Here's how the part is built. I have some questions about the finished solid (model axes, mm). A direction names the side the tool comes from. Coordinates: 2 decimals unless noted, no trailing zeros. Write each loop counter-clockwise with the first axis right and the second up, starting at its lowest first coordinate (ties: lowest second). Pieces come first, ordered by that corner, then holes.
Item 1: I want a section at A-A (x = 0). Please give me the cut outline in (y, z), and give its area (3 significant figures).
Item 2: I want a section at C-C (z = -19). Please give me the cut outline in (x, y), and give its area (3 significant figures).
Item 3: Please list where these lines run through material, in increasing order: line 1 (X direction, y = 1.2, z = 0); line 2 (X direction, y = 2.25, z = -4); line 3 (Y direction, x = -31, z = -31).
Item 4: I want a section at B-B (z = 0). Please give me the cut outline in (x, y), and give its area (3 significant figures).
Item 5: I'm going to push flat-ended pins straight in: P1, Ø5, axis at x = 28.5, z = 23, coming from the -Y side; P2, Ø2, axis at x = -18, y = 4, coming from the -Z side; P3, Ø1.5, axis at y = 1.5, z = -2, coming from the +X side. Where does each tip first touch, or does it pass through?
Item 6: For faces 1 (the face through (18.44, 3.166, -34.934)), 2 (the face through (19, 7.62, -33)), which set-ups out of +Z, -Z, +X, -X, +Y, -Y let a thin tool reach every point of the face, with its end or its side?
Item 7: I want a section at D-D (y = 6.25). Please give me the cut outline in (x, z), and give its area (3 significant figures).
from build123d import *

# Parameters (mm, degrees)
SKETCH1_R           = 44.45
SKETCH1_R_2         = 31.75
BOSS_EXTRUDE1_DEPTH = 2.54
CIRPATTERN1_COUNT   = 3


with BuildPart() as part:
    # Sketch1 → Boss-Extrude1 (new body)
    with BuildSketch(Plane(origin=(0, 0, 0), x_dir=(1, 0, 0), z_dir=(0, 1, 0))):
        with Locations(Location((0, 0, 0), (0, 0, 270))):
            Circle(SKETCH1_R)
        with Locations(Location((0, 0, 0), (0, 0, 270))):
            Circle(SKETCH1_R_2, mode=Mode.SUBTRACT)
    extrude(amount=BOSS_EXTRUDE1_DEPTH)

    # Sketch4 → Revolve1 (revolve)
    with BuildSketch(Plane.XY, mode=Mode.PRIVATE) as revolve1_sk:
        Polygon((-38.1, 2.54), (-38.1, 7.62), (-39.878, 7.62), (-40.132, 3.81), (-40.132, 2.54), align=None)
    revolve1 = revolve(revolve1_sk.sketch.rotate(Axis((-38.1, 2.54, 0), (0, 1, 0)), 270), axis=Axis((-38.1, 2.54, 0), (0, 1, 0)))

    # CirPattern1: Revolve1 ×3 about axis
    cirpattern1_axis = Axis((0, 0, 0), (0, 1, 0))
    for i in range(1, CIRPATTERN1_COUNT):
        add(revolve1.rotate(cirpattern1_axis, i * 360 / CIRPATTERN1_COUNT))


solid = part.part
Answer:
1. outline: (0, -44.45) - (2.54, -44.45) - (2.54, -31.75) - (0, -31.75) - close; (0, 31.75) - (2.54, 31.75) - (2.54, 44.45) - (0, 44.45) - close
1. area: 64.5 mm2
2. outline: (-40.18, 0) - (-25.44, 0) - (-25.44, 2.54) - (-40.18, 2.54) - close; (25.44, 0) - (40.18, 0) - (40.18, 2.54) - (25.44, 2.54) - close
2. area: 74.9 mm2
3. line 1: x = -44.45 to -31.75, 31.75 to 44.45
3. line 2: x = -44.27 to -31.5, 31.5 to 44.27
3. line 3: y = 0 to 2.54
4. outline: (-44.45, 0) - (-31.75, 0) - (-31.75, 2.54) - (-36.07, 2.54) - (-36.07, 3.81) - (-36.32, 7.62) - (-39.88, 7.62) - (-40.13, 3.81) - (-40.13, 2.54) - (-44.45, 2.54) - close; (31.75, 0) - (44.45, 0) - (44.45, 2.54) - (31.75, 2.54) - close
4. area: 84.2 mm2
5. P1: stops at y = 0
5. P2: passes through
5. P3: stops at x = 44.43
6. face 1: +Y
6. face 2: +Z, -Z, +X, -X, +Y
7. outline: circle Ø3.74 at (-38.1, 0); circle Ø3.74 at (19.05, -33); circle Ø3.74 at (19.05, 33)
7. area: 32.9 mm2
